Check sheet for the modelled part. Datum: model origin and axes. Units: mm. A direction names the side the tool comes from. Give positions to 0.01 mm unless a question says otherwise; leave off trailing zeros. Write each loop counter-clockwise with the first axis right and the second up, starting at its lowest first coordinate (ties: lowest second). Pieces come first, ordered by that corner, then holes. Notation, with made-up numbers: M -40,49 L -21,49 A26 ccw -21,87 Z; hole C 25.5,43.5 d7. An arc over 180 degrees is marked long. Use CSV: the item, a comma, the result in double quotes. Start each with the question number.
1. Cross-section at B-B, the plane x = 30. Enter the section's corners in (y, z) (3 decimals), and give its area (3 significant figures).
2. Mould release check, pull along X, two halves, no side actions. Record for faces 1 (the face through (0, -2, 18)), 2 (the face through (8, -2, 0)), 3 (the face through (14, 0, 18)): +X half, -X half, draft (parallel to the pull), parting line (faces both ways), or undercut.
3. Cross-section at A-A, the plane z = 8. Enter the section's corners in (x, y), and give its area (3 significant figures).
4. Cross-section at C-C, the plane y = 1.5. Enter the section's corners in (x, z).
5. Scan lines: line 1 (X direction, y = 1, z = 12); line 2 (X direction, y = -16, z = 13); line 3 (Y direction, x = 13, z = 28). Record each from-to range of solid material in increasing order.
6. Depth check by flat-ended pin: P1, Ø3, axis at y = -18.5, z = 22, coming from the +X side; P2, Ø15.5, axis at x = 25, z = 8, coming from the +Y side; P3, Ø8, axis at x = 26.5, z = 14.5, coming from the -Y side. Enter the tip coordinate at first touch or a pass-through.
7. Cross-section at D-D, the plane x = 26. Enter the section's corners in (y, z).
8. Access from +Z, -Z, +X, -X, +Y, -Y to the whole of each face (thin tool, end or side, straight path). Record for faces 4 (the face through (4.85, -7.01, 18.08)), 5 (the face through (5.01, 2.85, 18.08)), 6 (the face through (2, 16, 18)), 7 (the face through (20, -2, 13)), 8 (the face through (24.4, -8, 1.8)).
from build123d import *

# Parameters (mm, degrees)
SKETCH_R          = 1.5
PAD_DEPTH         = 4
PAD001_DEPTH      = 4
PAD001_DEPTH_BACK = 8
SKETCH002_W       = 35.656854
SKETCH002_H       = 50
PAD002_DEPTH      = 2
FILLET_R          = 10
FILLET001_R       = 3


with BuildPart() as part:
    # Sketch → Pad (new body)
    with BuildSketch(Plane.XZ):
        with BuildLine():
            ThreePointArc((20.757359, 12.242641), (25, 2), (29.242641, 12.242641))
            Line((30.656854, 13.656854), (29.242641, 12.242641))
            ThreePointArc((24.999973, 0), (32.391031, 4.93852), (30.656854, 13.656854))
            Line((0, 0), (24.999973, 0))
            Line((0, 35.656854), (0, 0))
            Line((0, 35.656854), (19, 35.656854))
            Line((19, 35.656854), (19, 13.656854))
            Line((19, 13.656854), (19.343146, 13.656854))
            Line((19.343146, 13.656854), (20.757359, 12.242641))
        make_face()
        with Locations((16, 32.656854)):
            Circle(SKETCH_R, mode=Mode.SUBTRACT)
        with Locations((16, 17.656854)):
            Circle(SKETCH_R, mode=Mode.SUBTRACT)
    extrude(amount=PAD_DEPTH)

    # Sketch001 → Pad001 (new body, two sides)
    with BuildSketch(Plane.XZ.offset(4)) as pad001_sk:
        with BuildLine():
            ThreePointArc((20.757359, 12.242641), (25, 2), (29.242641, 12.242641))
            Line((30.656854, 13.656854), (29.242641, 12.242641))
            ThreePointArc((19.343146, 13.656854), (25, 0), (30.656854, 13.656854))
            Line((20.757359, 12.242641), (19.343146, 13.656854))
        make_face()
    extrude(amount=PAD001_DEPTH)
    extrude(pad001_sk.sketch, amount=-PAD001_DEPTH_BACK)

    # Sketch002 → Pad002 (new body)
    with BuildSketch(Plane(origin=(0, 0, 0), x_dir=(0, 0, -1), z_dir=(-1, 0, 0))):
        with Locations((-17.828427, 2)):
            Rectangle(SKETCH002_W, SKETCH002_H)
    extrude(amount=-PAD002_DEPTH)

    # Fillet
    fillet_edges = [part.edges().sort_by_distance(p)[0] for p in [
        (2, -4, 17.828427),
        (2, 0, 17.828427),
    ]]
    fillet(fillet_edges, radius=FILLET_R)

    # Fillet001
    fillet001_edges = [part.edges().sort_by_distance(p)[0] for p in [
        (19, -2, 35.656854),
    ]]
    fillet(fillet001_edges, radius=FILLET001_R)


solid = part.part
Worked answers:
1,outline,"M -8,1.755 L 4,1.755 L 4,4.683 L -8,4.683 Z; M -8,11.317 L 4,11.317 L 4,13 L -8,13 Z"
1,area,"55.3 mm^2"
2,face 1,"-X half"
2,face 2,"draft"
2,face 3,"undercut"
3,outline,"M 0,-27 L 2,-27 L 2,-14 A10 cw 12,-4 L 17,-4 L 17,-8 L 19,-8 L 19,4 L 17,4 L 17,0 L 12,0 A10 cw 2,10 L 2,23 L 0,23 Z; M 31,-8 L 33,-8 L 33,4 L 31,4 Z"
3,area,"251 mm^2"
4,outline,"M 0,0 L 6.73,0 L 6.73,35.66 L 0,35.66 Z; M 19.34,13.66 A8 ccw long 30.66,13.66 L 29.24,12.24 A6 cw long 20.76,12.24 Z"
5,line 1,"x = 0 to 7.64, 18.07 to 20.53, 29.47 to 31.93"
5,line 2,"x = 0 to 2"
5,line 3,"y = -4 to 0"
6,P1,"stops at x = 2"
6,P2,"stops at y = 4"
6,P3,"stops at y = -8"
7,outline,"M -8,0.06 L 4,0.06 L 4,2.08 L -8,2.08 Z"
8,face 4,"+Z, -Z, -Y"
8,face 5,"+Z, -Z, +Y"
8,face 6,"+Z, -Z, +X, +Y"
8,face 7,"+Z, +Y, -Y"
8,face 8,"+Z, -Z, +X, -Y"
